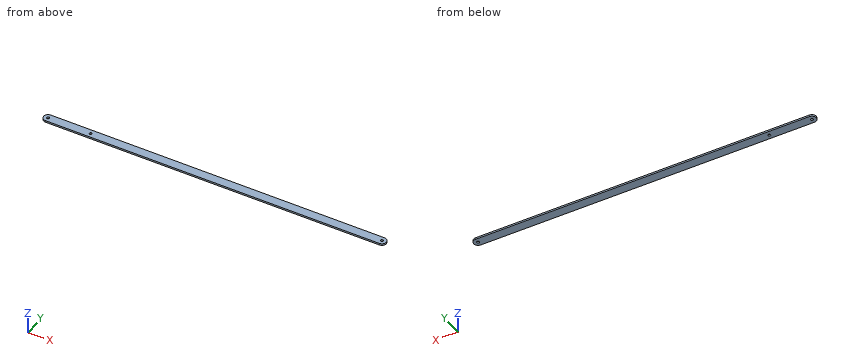
from build123d import *

# Parameters (mm, degrees)
SKETCH1_R           = 4.7625
BOSS_EXTRUDE1_DEPTH = 3.175
SKETCH2_R           = 4.7625
CUT_EXTRUDE1_DEPTH  = 614.01348986


with BuildPart() as part:
    # Sketch1 → Boss-Extrude1 (new, symmetric)
    with BuildSketch(Plane.XY):
        with BuildLine():
            Line((596.9, -15.875), (-596.9, -15.875))
            ThreePointArc((-596.9, -15.875), (-612.775, 0), (-596.9, 15.875))
            Line((-596.9, 15.875), (596.9, 15.875))
            ThreePointArc((596.9, 15.875), (612.775, 0), (596.9, -15.875))
        make_face()
        with Locations((-596.9, 0)):
            Circle(SKETCH1_R, mode=Mode.SUBTRACT)
        with Locations((596.9, 0)):
            Circle(SKETCH1_R, mode=Mode.SUBTRACT)
    extrude(amount=BOSS_EXTRUDE1_DEPTH, both=True)

    # Sketch2 → Cut-Extrude1 (cut, through all)
    with BuildSketch(Plane.XY.offset(3.175)):
        with Locations((-444.5, 0)):
            Circle(SKETCH2_R)
    extrude(amount=-CUT_EXTRUDE1_DEPTH, mode=Mode.SUBTRACT)


solid = part.part
Input: part model. Units: mm. Frame: model coordinates. Coordinates: 2 decimals unless noted, no trailing zeros. Order: outer loops, then holes, each group sorted by start corner. A loop starts at its lowest first (then second) coordinate and runs counter-clockwise, first axis right, second up. Notation, with made-up numbers: M -10.5,70 L 38.5,70 A14 ccw 38.5,92 Z; hole C 14.5,-20 d5. An arc over 180 degrees is marked long. Answer as CSV lines item,"result".
1. Section A-A (y = 0). Return the cut outline in (x, z) (1 decimal), then the cut area to 3 significant figures.
Reported:
outline,"M -612.8,-3.2 L -601.7,-3.2 L -601.7,3.2 L -612.8,3.2 Z; M -592.1,-3.2 L -449.3,-3.2 L -449.3,3.2 L -592.1,3.2 Z; M -439.7,-3.2 L 592.1,-3.2 L 592.1,3.2 L -439.7,3.2 Z; M 601.7,-3.2 L 612.8,-3.2 L 612.8,3.2 L 601.7,3.2 Z"
area,"7,600 mm2"
2. Material intervals for line 1 (X direction, y = 1, z = 1.75); line 2 (Y direction, x = -596.9, z = -1) (1 decimal); line 3 (X direction, y = -2.5, z = -2.5), sorted ascending. Write a range as from..to.
Reported:
line 1,"-612.74..-601.56, -592.24..-449.16, -439.84..592.24, 601.56..612.74"
line 2,"-15.9..-4.8, 4.8..15.9"
line 3,"-612.58..-600.95, -592.85..-448.55, -440.45..592.85, 600.95..612.58"
3. First-contact query: P1, Ø1.5, axis at y = -9.5, z = 1.5, coming from the -X side; P2, Ø5.5, axis at x = -596.9, y = 0, coming from the -Z side. Flat tips, straight axial feed; report the tip coordinate or a pass-through.
Reported:
P1,"x = -610.15"
P2,"through"
